Design review of the part built by this model. Coordinates are the model's own, in mm. Face numbers are marked on the shaded views. A direction names the side the tool comes from. Round coordinates to 2 decimals unless told otherwise and drop trailing zeros. Order: outer loops, then holes, each group sorted by start corner. A loop starts at its lowest first (then second) coordinate and runs counter-clockwise, first axis right, second up.
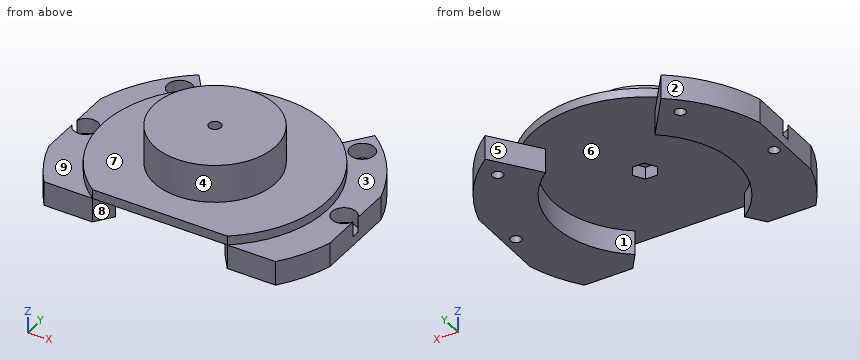
from build123d import *

# Parameters (mm, degrees)
SKETCH1_R           = 48.25
BOSS_EXTRUDE1_DEPTH = 8
SKETCH2_W           = 17.162038191
SKETCH2_H           = 56.822210482
SKETCH2_W_2         = 16.152506533
SKETCH2_H_2         = 65.186901365
CUT_EXTRUDE1_DEPTH  = 8
SKETCH3_R           = 30
CUT_EXTRUDE2_DEPTH  = 8
SKETCH4_R           = 1.75
CUT_EXTRUDE3_DEPTH  = 10
CIRPATTERN1_COUNT   = 8
CUT_EXTRUDE4_DEPTH  = 10
CIRPATTERN2_COUNT   = 2
SKETCH10_R          = 4
CUT_EXTRUDE6_DEPTH  = 5
SKETCH11_R          = 37
BOSS_EXTRUDE2_DEPTH = 3
SKETCH12_R          = 20
BOSS_EXTRUDE3_DEPTH = 12.5
SKETCH13_R          = 2
CUT_EXTRUDE8_DEPTH  = 38
CUT_EXTRUDE9_DEPTH  = 4
SKETCH15_W          = 91.603546033
SKETCH15_H          = 22.115690979
CUT_EXTRUDE10_DEPTH = 34
SKETCH9_R           = 4
CUT_EXTRUDE11_DEPTH = 5
SKETCH16_W          = 4.965700005
SKETCH16_H          = 2.207169135
SKETCH16_W_2        = 4.07415349
BOSS_EXTRUDE4_DEPTH = 8


with BuildPart() as part:
    # Sketch1 → Boss-Extrude1 (new body)
    with BuildSketch(Plane.XY):
        Circle(SKETCH1_R)
    extrude(amount=-BOSS_EXTRUDE1_DEPTH)

    # Sketch2 → Cut-Extrude1 (cut)
    with BuildSketch(Plane.XY):
        with Locations((-54.831019095, 0)):
            Rectangle(SKETCH2_W, SKETCH2_H)
        with Locations((54.326253267, -4.182345442)):
            Rectangle(SKETCH2_W_2, SKETCH2_H_2)
    extrude(amount=-CUT_EXTRUDE1_DEPTH, mode=Mode.SUBTRACT)

    # Sketch3 → Cut-Extrude2 (cut)
    with BuildSketch(Plane.XY):
        Circle(SKETCH3_R)
    extrude(amount=-CUT_EXTRUDE2_DEPTH, mode=Mode.SUBTRACT)

    # Sketch4 → Cut-Extrude3 (cut)
    with BuildSketch(Plane.XY):
        with Locations((-42.5, 0)):
            Circle(SKETCH4_R)
    cut_extrude3 = extrude(amount=-CUT_EXTRUDE3_DEPTH, mode=Mode.SUBTRACT)

    # CirPattern1: Cut-Extrude3 ×8 about axis
    cirpattern1_axis = Axis((0, 0, 0), (0, 0, 1))
    for i in range(1, CIRPATTERN1_COUNT):
        add(cut_extrude3.rotate(cirpattern1_axis, i * 360 / CIRPATTERN1_COUNT), mode=Mode.SUBTRACT)

    # Sketch8 → Cut-Extrude4 (cut)
    with BuildSketch(Plane.XY):
        with BuildLine():
            Line((-28.959547499, 38.59283753), (0, 0))
            Line((0, 0), (28.959547499, 38.59283753))
            ThreePointArc((28.959547499, 38.59283753), (0, 48.25), (-28.959547499, 38.59283753))
        make_face()
    cut_extrude4 = extrude(amount=-CUT_EXTRUDE4_DEPTH, mode=Mode.SUBTRACT)

    # CirPattern2: Cut-Extrude4 ×2 about axis
    cirpattern2_axis = Axis((0, 0, 0), (0, 0, 1))
    for i in range(1, CIRPATTERN2_COUNT):
        add(cut_extrude4.rotate(cirpattern2_axis, i * 360 / CIRPATTERN2_COUNT), mode=Mode.SUBTRACT)

    # Sketch10 → Cut-Extrude6 (cut)
    with BuildSketch(Plane.XY):
        with Locations((42.5, 0)):
            Circle(SKETCH10_R)
        with Locations((30.0520382, 30.0520382)):
            Circle(SKETCH10_R)
    extrude(amount=-CUT_EXTRUDE6_DEPTH, mode=Mode.SUBTRACT)

    # Sketch11 → Boss-Extrude2 (add)
    with BuildSketch(Plane.XY):
        with Locations(Location((0, 0, 0), (0, 0, 126.884070759))):
            Circle(SKETCH11_R)
    extrude(amount=BOSS_EXTRUDE2_DEPTH)

    # Sketch12 → Boss-Extrude3 (add)
    with BuildSketch(Plane.XY.offset(3)):
        Circle(SKETCH12_R)
    extrude(amount=BOSS_EXTRUDE3_DEPTH)

    # Sketch13 → Cut-Extrude8 (cut)
    with BuildSketch(Plane.XY.offset(15.5)):
        Circle(SKETCH13_R)
    extrude(amount=-CUT_EXTRUDE8_DEPTH, mode=Mode.SUBTRACT)

    # Sketch14 → Cut-Extrude9 (cut)
    with BuildSketch(Plane(origin=(0, 0, 0), x_dir=(-1, 0, 0), z_dir=(0, 0, -1))):
        Polygon((-2.020725942, -3.5), (2.020725942, -3.5), (4.041451884, 0), (2.020725942, 3.5), (-2.020725942, 3.5), (-4.041451884, 0), align=None)
    extrude(amount=-CUT_EXTRUDE9_DEPTH, mode=Mode.SUBTRACT)

    # Sketch15 → Cut-Extrude10 (cut)
    with BuildSketch(Plane(origin=(0, 0, -8), x_dir=(-1, 0, 0), z_dir=(0, 0, -1))):
        with Locations((2.592277623, -40.652353026)):
            Rectangle(SKETCH15_W, SKETCH15_H)
    extrude(amount=-CUT_EXTRUDE10_DEPTH, mode=Mode.SUBTRACT)

    # Sketch9 → Cut-Extrude11 (cut)
    with BuildSketch(Plane.XY):
        with Locations((-42.5, 0)):
            Circle(SKETCH9_R)
        with Locations((-30.0520382, 30.0520382)):
            Circle(SKETCH9_R)
    extrude(amount=-CUT_EXTRUDE11_DEPTH, mode=Mode.SUBTRACT)

    # Sketch16 → Boss-Extrude4 (add)
    with BuildSketch(Plane.XY):
        with Locations((-30.845756565, -28.490922969)):
            Rectangle(SKETCH16_W, SKETCH16_H)
        with Locations((29.704093094, -28.490922969)):
            Rectangle(SKETCH16_W_2, SKETCH16_H)
    extrude(amount=-BOSS_EXTRUDE4_DEPTH)


solid = part.part
1) The part is to be moulded in two halves that separate along Y. For the marked faces 1, 2, 3 and 4, say which applies: released by +Y, released by -Y, zero draft, split by the parting line, or undercut.
Results:
face 1: undercut
face 2: released by +Y
face 3: zero draft
face 4: split by the parting line
2) Take a section at A-A on x = 0. Give the boundary of the cut face in (y, z).
Results:
outline: (-29.59, 0) - (-3.5, 0) - (-3.5, 4) - (-2, 4) - (-2, 15.5) - (-20, 15.5) - (-20, 3) - (-29.59, 3) - close; (2, 4) - (3.5, 4) - (3.5, 0) - (37, 0) - (37, 3) - (20, 3) - (20, 15.5) - (2, 15.5) - close
3) For the marked faces 5, 6, 7, 8 and 9, list the 3-axis set-ups (+Z, -Z, +X, -X, +Y, -Y) from which the entire face can be reached by the end or side of a thin tool; tool diameter is ignored.
Results:
face 5: -Z, +Y
face 6: -Z
face 7: +Z
face 8: -Z, -Y
face 9: +Z, -X
4) Take a section at C-C on y = -19. Give the boundary of the cut face in (x, z) (3 decimals), plus the area to 3 significant figures.
Results:
outline: (-44.352, -8) - (-23.216, -8) - (-23.216, 0) - (23.216, 0) - (23.216, -8) - (44.352, -8) - (44.352, 0) - (31.749, 0) - (31.749, 3) - (6.245, 3) - (6.245, 15.5) - (-6.245, 15.5) - (-6.245, 3) - (-31.749, 3) - (-31.749, 0) - (-44.352, 0) - close
area: 685 mm2
5) To check wall thickness, follow line 1 along Y through (x, z) = (27.5, -3.25); line 2 along X through (y, z) = (0, -1.85); line 3 along Z through (x, y) = (-16, 15.5). State the ranges of each line that lie inside material, in increasing order.
Results:
line 1: y = -29.59 to -11.99, 11.99 to 26.97, 33.13 to 36.65
line 2: x = -38.5 to -30, 30 to 38.5
line 3: z = 0 to 3
6) Clearance check with flat-ended pins moving along their axes: P1, Ø2, axis at y = 28, z = -2, coming from the -X side; P2, Ø6.5, axis at x = -29.5, y = 28, coming from the +Z side; P3, Ø5, axis at x = 30.05, y = 30.05, coming from the +Z side; P4, Ø5, axis at x = -24, z = 12.5, coming from the +Y side. State where each tip first meets the part, or that it passes through.
Results:
P1: stops at x = -39.99
P2: stops at z = 0
P3: stops at z = -5
P4: passes through
7) Take a section at B-B on z = 1. Give the boundary of the cut face in (x, y).
Results:
outline: (-22.21, -29.59) - (22.21, -29.59) arc R37 ccw (long way) to start; hole (-4.04, 0) - (-2.02, -3.5) - (2.02, -3.5) - (4.04, 0) - (2.02, 3.5) - (-2.02, 3.5) - close
8) Take a section at D-D on x = -42.5. Give the boundary of the cut face in (y, z).
Results:
outline: (-22.84, -8) - (-1.75, -8) - (-1.75, -5) - (-4, -5) - (-4, 0) - (-22.84, 0) - close; (1.75, -8) - (22.84, -8) - (22.84, 0) - (4, 0) - (4, -5) - (1.75, -5) - close
